```python
from build123d import *

# Parameters (mm, degrees)
EXTRUDE_1_DEPTH     = 30
EXTRUDE_2_DEPTH     = 101.4074
CUT_EXTRUDE_2_DEPTH = 140.67269183
CUT_EXTRUDE_3_DEPTH = 134.91587226
SKETCH_10_W         = 30
SKETCH_10_H         = 25
CUT_EXTRUDE_6_DEPTH = 4
SKETCH_11_W         = 30
SKETCH_11_H         = 25
CUT_EXTRUDE_7_DEPTH = 4
SKETCH_13_R         = 2.15
CUT_EXTRUDE_8_DEPTH = 139.001669711
SKETCH_14_R         = 5
CUT_EXTRUDE_9_DEPTH = 40


with BuildPart() as part:
    # 草图2 → 凸台-拉伸1 (new body)
    with BuildSketch(Plane(origin=(0, 0, 0), x_dir=(1, 0, 0), z_dir=(0, 1, 0))):
        Polygon((0, 0), (71.407400337, 50), (71.407400337, 75), (101.407400337, 75), (101.407400337, 30), (40, 0), align=None)
    extrude(amount=EXTRUDE_1_DEPTH)

    # 草图4 → 凸台-拉伸2 (add, through all)
    with BuildSketch(Plane(origin=(101.407400337, 0, 0), x_dir=(0, 0, -1), z_dir=(1, 0, 0))):
        Polygon((0, 30), (30, 45), (75, 45), (75, 30), align=None)
        Polygon((0, 0), (75, 0), (75, -15), (30, -15), align=None)
    extrude(amount=-EXTRUDE_2_DEPTH)

    # 草图5 → 切除-拉伸2 (cut, through all)
    with BuildSketch(Plane.XZ.offset(15)):
        Polygon((40, 0), (101.407400337, 0), (101.407400337, -30), align=None)
        Polygon((0, 0), (0, -75), (71.407400337, -75), (71.407400337, -50), align=None)
    extrude(amount=-CUT_EXTRUDE_2_DEPTH, mode=Mode.SUBTRACT)

    # 草图6 → 切除-拉伸3 (cut, through all)
    with BuildSketch(Plane(origin=(0, 0, 0), x_dir=(-0.8191520442889949, 0, 0.5735764363510418), z_dir=(-0.5735764363510418, 0, -0.8191520442889949))):
        Polygon((0, 21), (-26.151701934, 37.5), (0, 30), align=None)
        Polygon((0, 0), (-26.151701934, -7.5), (0, 9), align=None)
    extrude(amount=-CUT_EXTRUDE_3_DEPTH, mode=Mode.SUBTRACT)

    # 草图10 → 切除-拉伸6 (cut)
    with BuildSketch(Plane.XZ.offset(15)):
        with Locations((86.407400337, -62.5)):
            Rectangle(SKETCH_10_W, SKETCH_10_H)
    extrude(amount=-CUT_EXTRUDE_6_DEPTH, mode=Mode.SUBTRACT)

    # 草图11 → 切除-拉伸7 (cut)
    with BuildSketch(Plane(origin=(0, 45, 0), x_dir=(1, 0, 0), z_dir=(0, 1, 0))):
        with Locations((86.407400337, 62.5)):
            Rectangle(SKETCH_11_W, SKETCH_11_H)
    extrude(amount=-CUT_EXTRUDE_7_DEPTH, mode=Mode.SUBTRACT)

    # 草图13 → 切除-拉伸8 (cut, through all)
    with BuildSketch(Plane(origin=(0, 41, 0), x_dir=(1, 0, 0), z_dir=(0, 1, 0))):
        with Locations(Location((78.907400337, 62.5, 0), (0, 0, 270))):
            Circle(SKETCH_13_R)
        with Locations(Location((93.907400337, 62.5, 0), (0, 0, 270))):
            Circle(SKETCH_13_R)
    extrude(amount=-CUT_EXTRUDE_8_DEPTH, mode=Mode.SUBTRACT)

    # 草图14 → 切除-拉伸9 (cut)
    with BuildSketch(Plane(origin=(0, 0, -75), x_dir=(-1, 0, 0), z_dir=(0, 0, -1))):
        with Locations((-86.407400337, 15)):
            Circle(SKETCH_14_R)
    extrude(amount=-CUT_EXTRUDE_9_DEPTH, mode=Mode.SUBTRACT)


solid = part.part
```
For this review, take the finished solid that the model builds, in its own axes (mm). A direction names the side the tool comes from. Give positions to 0.01 mm unless a question says otherwise; leave off trailing zeros. Write each loop counter-clockwise with the first axis right and the second up, starting at its lowest first coordinate (ties: lowest second). Pieces come first, ordered by that corner, then holes. Notation, with made-up numbers: M 41,-20 L 70,-20 A15 cw 70,-14 Z; hole C 87,43 d6. An arc over 180 degrees is marked long. Answer as CSV lines item,"result".
1. For faces 4 (the flat face through (86, -13, -50)), 5 (the flat face through (86, 41, -63)), 6 (the flat face through (79, -15, -40)), 7 (the flat face through (71.407, 15, -63)), 8 (the flat face through (86, 15, -35)), list the 3-axis set-ups (+Z, -Z, +X, -X, +Y, -Y) from which the entire face can be reached by the end or side of a thin tool; tool diameter is ignored.
Findings:
face 4,"-Z, +X, -X, -Y"
face 5,"-Z, +X, -X, +Y"
face 6,"+Z, -Z, +X, -X, -Y"
face 7,"-Z, -X, +Y, -Y"
face 8,"-Z"
2. Consider section D-D, the plane y = 25. Write out the cut boundary in (x, z).
Findings:
outline,"M 5.19,-3.64 L 71.41,-50 L 71.41,-75 L 101.41,-75 L 101.41,-30 L 40,0 L 7.74,0 Z; hole C 78.91,-62.5 d4.3; hole C 93.91,-62.5 d4.3"
3. For pin 1 (2 mm diameter, centred on x = 68, z = -14.5, fed in from +Y); pin 2 (3.5 mm diameter, centred on x = 93.91, z = -62.5, fed in from +Y); pin 3 (2 mm diameter, centred on x = 59, y = 1.5, fed in from +Z); pin 4 (8 mm diameter, centred on x = 88, y = 13.5, fed in from -Z), all flat-tipped, find the tip position at first contact; note any pin that passes through.
Findings:
pin 1,"stops at y = 37.75"
pin 2,"passes through"
pin 3,"stops at z = -8.79"
pin 4,"stops at z = -75"
4. Wall thickness on line 1 (X direction, y = 19, z = -62); line 2 (Y direction, x = 74, z = -63); line 3 (Y direction, x = 90.5, z = -56): over which ranges is each line inside the solid? List them lowest first.
Findings:
line 1,"x = 71.41 to 76.82, 81 to 83.41, 89.41 to 91.82, 96 to 101.41"
line 2,"y = -11 to 41"
line 3,"y = -11 to 12.13, 17.87 to 41"
5. Draft analysis for pull direction X (two halves, no side actions). For faces 1 (the flat face through (13.049, 0.635, -4.48)), 2 (the cylindrical face through (95.36, 15.364, -64.085)), 3 (the flat face through (101.407, 15, -53)), state which applies: +X half, -X half, draft (parallel to the pull), parting line (faces both ways), or undercut.
Findings:
face 1,"-X half"
face 2,"undercut"
face 3,"+X half"
6. Consider section A-A, the plane z = -62.5. Write out the cut boundary in (x, y), then the cut area to 3 significant figures.
Findings:
outline,"M 71.41,-11 L 76.76,-11 L 76.76,41 L 71.41,41 Z; M 81.06,-11 L 91.76,-11 L 91.76,41 L 81.06,41 Z; M 96.06,-11 L 101.41,-11 L 101.41,41 L 96.06,41 Z; hole C 86.41,15 d10"
area,"1,030 mm2"
7. Consider section C-C, the plane x = 75. Write out the cut boundary in (y, z), then the cut area to 3 significant figures.
Findings:
outline,"M -15,-50 L -11,-50 L -11,-75 L 41,-75 L 41,-50 L 45,-50 L 45,-30 L 38.55,-17.1 L -8.55,-17.1 L -15,-30 Z"
area,"3,190 mm2"
8. Consider section B-B, the plane y = 15. Write out the cut boundary in (x, z).
Findings:
outline,"M 0,0 L 71.41,-50 L 71.41,-75 L 81.41,-75 L 81.41,-35 L 91.41,-35 L 91.41,-75 L 101.41,-75 L 101.41,-30 L 40,0 Z; hole C 78.91,-62.5 d4.3; hole C 93.91,-62.5 d4.3"
